Read the model definition and answer for the solid it produces. Units are mm, in the model's axes. Round coordinates to 2 decimals unless told otherwise and drop trailing zeros. Order: outer loops, then holes, each group sorted by start corner. A loop starts at its lowest first (then second) coordinate and runs counter-clockwise, first axis right, second up. Notation, with made-up numbers: (70.5, 71.25) - (80.5, 71.25) arc R9 ccw to (80.5, 76.25) - close; hole circle Ø9 at (22.5, -15.75). An arc over 180 degrees is marked (long way). Put each result on its own line as item: value. Start each with the question number.
Q1. Find the intervals of material crossed by line 1 along X through (y, z) = (2.15, 137.5); line 2 along Z through (x, y) = (81.5, 2.2); line 3 along X through (y, z) = (1.9, 134), in increasing order. Write a range as from..to.
Q2. Section A-A on x = -137.5 is taken. Give the vertices of the cut face in (y, z) (3 decimals).
Q3. Section B-B on y = 1.4 is taken. Give the vertices of the cut face in (x, z), then the cut area to 3 significant figures.
Q4. This flat-tipped pin is pushed along its axis until it touches: pin 1 Ø13 at (x, z) = (-137.5, 137.5) entering from +Y (3 decimals). Where does it stop, or does it pass through?
Q5. For a pull along Z with two mould halves and no side action, classify faces 1 (the face through (142.4, 1.6, -142.5)), 2 (the face through (-2, 0, -2)), 3 (the face through (132.6, 1.6, -132.5)) as pulls with the +Z half, pulls with the -Z half, needs draft (parallel to the pull), parting line crosses it, or undercut.
Q6. Section C-C on z = 137.5 is taken. Give the vertices of the cut face in (x, y) (3 decimals).
from build123d import *

# Parameters (mm, degrees)
SKETCH1_W           = 300
SKETCH1_H           = 300
BOSS_EXTRUDE1_DEPTH = 3.175
SKETCH2_R           = 5
CUT_EXTRUDE1_DEPTH  = 213.155793286
SKETCH3_W           = 34.06
SKETCH3_H           = 46.67
CUT_EXTRUDE2_DEPTH  = 213.155793286


with BuildPart() as part:
    # Sketch1 → Boss-Extrude1 (new body)
    with BuildSketch(Plane(origin=(0, 0, 0), x_dir=(1, 0, 0), z_dir=(0, 1, 0))):
        Rectangle(SKETCH1_W, SKETCH1_H)
    extrude(amount=BOSS_EXTRUDE1_DEPTH)

    # Sketch2 → Cut-Extrude1 (cut, through all)
    with BuildSketch(Plane(origin=(0, 3.175, 0), x_dir=(1, 0, 0), z_dir=(0, 1, 0))):
        with Locations(Location((-137.5, -137.5, 0), (0, 0, 270))):
            Circle(SKETCH2_R)
        with BuildLine():
            Line((142.449747468, 135.378679656), (139.621320344, 132.550252532))
            ThreePointArc((139.621320344, 132.550252532), (132.550252532, 132.550252532), (132.550252532, 139.621320344))
            Line((132.550252532, 139.621320344), (135.378679656, 142.449747468))
            ThreePointArc((135.378679656, 142.449747468), (142.449747468, 142.449747468), (142.449747468, 135.378679656))
        make_face()
    extrude(amount=-CUT_EXTRUDE1_DEPTH, mode=Mode.SUBTRACT)

    # Sketch3 → Cut-Extrude2 (cut, through all)
    with BuildSketch(Plane(origin=(0, 3.175, 0), x_dir=(1, 0, 0), z_dir=(0, 1, 0))):
        with Locations((74.716012632, 31.592141137)):
            Rectangle(SKETCH3_W, SKETCH3_H)
    extrude(amount=-CUT_EXTRUDE2_DEPTH, mode=Mode.SUBTRACT)


solid = part.part
Findings:
1. line 1: -150..-142.5, -132.5..150
1. line 2: -150..-54.93, -8.26..150
1. line 3: -150..-141.07, -133.93..150
2. outline: (0, -150) - (3.175, -150) - (3.175, 132.5) - (0, 132.5) - close; (0, 142.5) - (3.175, 142.5) - (3.175, 150) - (0, 150) - close
3. outline: (-150, -150) - (150, -150) - (150, 150) - (-150, 150) - close; hole circle Ø10 at (-137.5, 137.5); hole (57.69, -54.93) - (91.75, -54.93) - (91.75, -8.26) - (57.69, -8.26) - close; hole (132.55, -139.62) - (135.38, -142.45) arc R5 ccw to (142.45, -135.38) - (139.62, -132.55) arc R5 ccw to start
3. area: 88,200 mm2
4. pin 1: y = 3.175
5. face 1: undercut
5. face 2: needs draft
5. face 3: undercut
6. outline: (-150, 0) - (-142.5, 0) - (-142.5, 3.175) - (-150, 3.175) - close; (-132.5, 0) - (150, 0) - (150, 3.175) - (-132.5, 3.175) - close
